Could you check a few things on this model? Use its own coordinates, in mm. Face numbers are marked on the shaded views. A direction names the side the tool comes from. Give positions to 0.01 mm unless a question says otherwise; leave off trailing zeros. Order: outer loops, then holes, each group sorted by start corner. A loop starts at its lowest first (then second) coordinate and runs counter-clockwise, first axis right, second up. Notation, with made-up numbers: (17, 9.5) - (27, 9.5) arc R15 ccw to (27, 28.5) - close; hole circle Ø8 at (29, 84). An arc over 180 degrees is marked (long way). One line per question, with ' | ' between items. Start each with the question number.
1. I need wall thicknesses on probe 1 along Y at (x, z) = (9.25, -2.25); probe 2 along X at (y, z) = (5.25, 7.5); probe 3 along X at (y, z) = (1.2, 0) (3 decimals). Which ranges of each line are inside material? Lowest first, please. Write a range as from..to.
2. Imagine slicing it at C-C (y = 17.75). Please give me the cut outline in (x, z), and give its area (4 significant figures).
3. Imagine slicing it at D-D (x = 7.75). Please give me the cut outline in (y, z).
4. Which directions (+Z, -Z, +X, -X, +Y, -Y) give clear straight access to the entire face, cutting with the end or side of a thin tool? Please do the marked faces 4, 5, 6 and 7.
5. Imagine slicing it at A-A (x = 5.5). Please give me the cut outline in (y, z).
6. For P1, Ø0.8, axis at x = 9.5, y = 7.5, coming from the +Z side; P2, Ø0.9, axis at y = 4.5, z = 9, coming from the +X side; P3, Ø3.5, axis at x = 0, z = 0, coming from the +Y side, each with a flat end and sliding along its axis, tell me the tip position at first contact or that it passes through.
7. If we mould it in two halves opening along Z, with no side actions, what happens to the marked faces 1, 2 and 3? For each: released by +Z, released by -Z, zero draft, split by the parting line, or undercut.
8. Imagine slicing it at B-B (z = 9.25). Please give me the cut outline in (x, y), and give its area (3 significant figures).
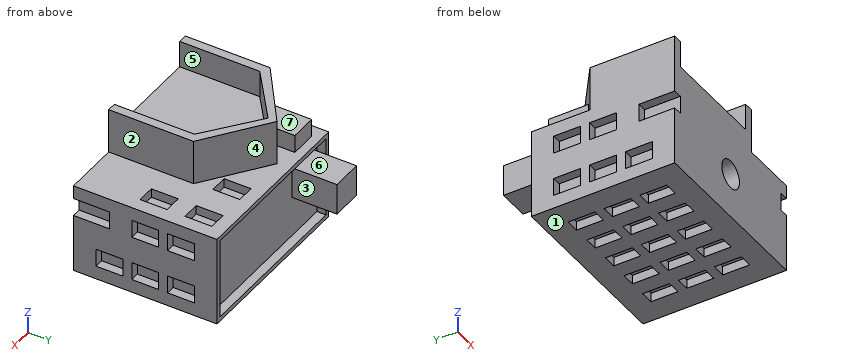
```python
from build123d import *

# Parameters (mm, degrees)
CROQUIS1_W              = 20
CROQUIS1_H              = 10
SALIENTE_EXTRUIR1_DEPTH = 15
SALIENTE_EXTRUIR2_DEPTH = 5
SALIENTE_EXTRUIR3_DEPTH = 2
CROQUIS4_W              = 19
CROQUIS4_H              = 9
SALIENTE_EXTRUIR4_DEPTH = 1
CROQUIS4_3_W            = 3.5
CROQUIS4_3_H            = 3.5
SALIENTE_EXTRUIR5_DEPTH = 5
CROQUIS5_R              = 1.575
CORTAR_EXTRUIR1_DEPTH   = 2.5
CORTAR_EXTRUIR2_DEPTH   = 3
CROQUIS7_W              = 2
CROQUIS7_H              = 3
CORTAR_EXTRUIR3_DEPTH   = 1
CROQUIS8_W              = 2
CROQUIS8_H              = 4
CROQUIS8_H_2            = 3
CORTAR_EXTRUIR4_DEPTH   = 1
CROQUIS9_W              = 1.5
CROQUIS9_H              = 3
CORTAR_EXTRUIR5_DEPTH   = 1


with BuildPart() as part:
    # Croquis1 → Saliente-Extruir1 (new body)
    with BuildSketch(Plane(origin=(0, 0, 0), x_dir=(1, 0, 0), z_dir=(0, 1, 0))):
        Rectangle(CROQUIS1_W, CROQUIS1_H)
    extrude(amount=SALIENTE_EXTRUIR1_DEPTH)

    # Croquis2 → Saliente-Extruir2 (add)
    with BuildSketch(Plane.XY.offset(5)):
        Polygon((-10, 0), (3.69887005, 0), (3.69887005, 9.460087219), (-3.150564975, 14.5), (-10, 9.460087219), align=None)
    extrude(amount=SALIENTE_EXTRUIR2_DEPTH)

    # Croquis3 → Saliente-Extruir3 (add)
    with BuildSketch(Plane.XY.offset(5)):
        Polygon((-8.552244838, 10.525366285), (-8.552244838, 15), (-5.552244838, 15), (-5.552244838, 12.732809422), align=None)
    extrude(amount=SALIENTE_EXTRUIR3_DEPTH)

    # Croquis4 → Saliente-Extruir4 (add)
    with BuildSketch(Plane(origin=(0, 15, 0), x_dir=(1, 0, 0), z_dir=(0, 1, 0))):
        Polygon((-10, 4.5), (-10, -4.5), (-10, -5), (-9.5, -5), (9.5, -5), (10, -5), (10, -4.5), (10, 4.5), (10, 5), (9.5, 5), (-9.5, 5), (-10, 5), align=None)
        Rectangle(CROQUIS4_W, CROQUIS4_H, mode=Mode.SUBTRACT)
    extrude(amount=SALIENTE_EXTRUIR4_DEPTH)

    # Croquis4_3 → Saliente-Extruir5 (add)
    with BuildSketch(Plane(origin=(0, 15, 0), x_dir=(1, 0, 0), z_dir=(0, 1, 0))):
        with Locations((-6.802244838, -1.75)):
            Rectangle(CROQUIS4_3_W, CROQUIS4_3_H)
    extrude(amount=SALIENTE_EXTRUIR5_DEPTH)

    # Croquis5 → Cortar-Extruir1 (cut)
    with BuildSketch(Plane.XZ):
        with Locations(Location((0, 0, 0), (0, 0, 270))):
            Circle(CROQUIS5_R)
    extrude(amount=-CORTAR_EXTRUIR1_DEPTH, mode=Mode.SUBTRACT)

    # Croquis6 → Cortar-Extruir2 (cut)
    with BuildSketch(Plane.XY.offset(10)):
        Polygon((-9, 8.935724798), (-9, 0), (2.69887005, 0), (2.69887005, 8.933581491), (-3.150564975, 13.5), align=None)
    extrude(amount=-CORTAR_EXTRUIR2_DEPTH, mode=Mode.SUBTRACT)

    # Croquis7 → Cortar-Extruir3 (cut)
    with BuildSketch(Plane.XY.offset(5)):
        with Locations((2.5, 12.998129378)):
            Rectangle(CROQUIS7_W, CROQUIS7_H)
        with Locations((7.5, 12.998129378)):
            Rectangle(CROQUIS7_W, CROQUIS7_H)
        with Locations((7.5, 7.998129378)):
            Rectangle(CROQUIS7_W, CROQUIS7_H)
    extrude(amount=-CORTAR_EXTRUIR3_DEPTH, mode=Mode.SUBTRACT)

    # Croquis8 → Cortar-Extruir4 (cut)
    with BuildSketch(Plane.ZY.offset(10)):
        with Locations((2.5, 2)):
            Rectangle(CROQUIS8_W, CROQUIS8_H)
        with Locations((-2.5, 4)):
            Rectangle(CROQUIS8_W, CROQUIS8_H_2)
        with Locations((-2.5, 8)):
            Rectangle(CROQUIS8_W, CROQUIS8_H_2)
        with Locations((-2.5, 12)):
            Rectangle(CROQUIS8_W, CROQUIS8_H_2)
        with Locations((2.5, 12)):
            Rectangle(CROQUIS8_W, CROQUIS8_H_2)
        with Locations((2.5, 8)):
            Rectangle(CROQUIS8_W, CROQUIS8_H_2)
    cortar_extruir4 = extrude(amount=-CORTAR_EXTRUIR4_DEPTH, mode=Mode.SUBTRACT)

    # Croquis9 → Cortar-Extruir5 (cut)
    with BuildSketch(Plane(origin=(0, 0, -5), x_dir=(-1, 0, 0), z_dir=(0, 0, -1))):
        with Locations((-3.336666667, 4)):
            Rectangle(CROQUIS9_W, CROQUIS9_H)
        with Locations((-6.666666667, 4)):
            Rectangle(CROQUIS9_W, CROQUIS9_H)
        with Locations((-0.006666667, 4)):
            Rectangle(CROQUIS9_W, CROQUIS9_H)
        with Locations((3.323333333, 4)):
            Rectangle(CROQUIS9_W, CROQUIS9_H)
        with Locations((6.653333333, 4)):
            Rectangle(CROQUIS9_W, CROQUIS9_H)
        with Locations((-3.336666667, 8)):
            Rectangle(CROQUIS9_W, CROQUIS9_H)
        with Locations((-0.006666667, 8)):
            Rectangle(CROQUIS9_W, CROQUIS9_H)
        with Locations((3.323333333, 8)):
            Rectangle(CROQUIS9_W, CROQUIS9_H)
        with Locations((6.653333333, 8)):
            Rectangle(CROQUIS9_W, CROQUIS9_H)
        with Locations((-3.336666667, 12)):
            Rectangle(CROQUIS9_W, CROQUIS9_H)
        with Locations((-0.006666667, 12)):
            Rectangle(CROQUIS9_W, CROQUIS9_H)
        with Locations((3.323333333, 12)):
            Rectangle(CROQUIS9_W, CROQUIS9_H)
        with Locations((6.653333333, 12)):
            Rectangle(CROQUIS9_W, CROQUIS9_H)
        with Locations((-6.666666667, 8)):
            Rectangle(CROQUIS9_W, CROQUIS9_H)
        with Locations((-6.666666667, 12)):
            Rectangle(CROQUIS9_W, CROQUIS9_H)
    extrude(amount=-CORTAR_EXTRUIR5_DEPTH, mode=Mode.SUBTRACT)

    # Simetr_a1: Cortar-Extruir4 across plane
    add(cortar_extruir4.mirror(Plane(origin=(0, 0, 0), x_dir=(0, 0, 1), z_dir=(1, 0, 0))), mode=Mode.SUBTRACT)


solid = part.part
```
Results found:
1) probe 1: y = 0..2.5, 5.5..6.5, 9.5..10.5, 13.5..15 | probe 2: x = -10..-9, 2.7..3.7 | probe 3: x = -10..-1.575, 1.575..10
2) outline: (-8.55, 0) - (-5.05, 0) - (-5.05, 3.5) - (-8.55, 3.5) - close | area: 12.25 mm2
3) outline: (0, -5) - (16, -5) - (16, -4.5) - (15, -4.5) - (15, 4.5) - (16, 4.5) - (16, 5) - (14.5, 5) - (14.5, 4) - (11.5, 4) - (11.5, 5) - (9.5, 5) - (9.5, 4) - (6.5, 4) - (6.5, 5) - (0, 5) - close
4) face 4: +Z, +X, +Y | face 5: +Z, -Y | face 6: +Y | face 7: +Z, -X, +Y
5) outline: (0, -5) - (16, -5) - (16, -4.5) - (15, -4.5) - (15, 4.5) - (16, 4.5) - (16, 5) - (0, 5) - close
6) P1: stops at z = 5 | P2: stops at x = 3.7 | P3: stops at y = 15
7) face 1: released by -Z | face 2: zero draft | face 3: undercut
8) outline: (-10, 0) - (-9, 0) - (-9, 8.94) - (-3.15, 13.5) - (2.7, 8.93) - (2.7, 0) - (3.7, 0) - (3.7, 9.46) - (-3.15, 14.5) - (-10, 9.46) - close | area: 32.9 mm2
